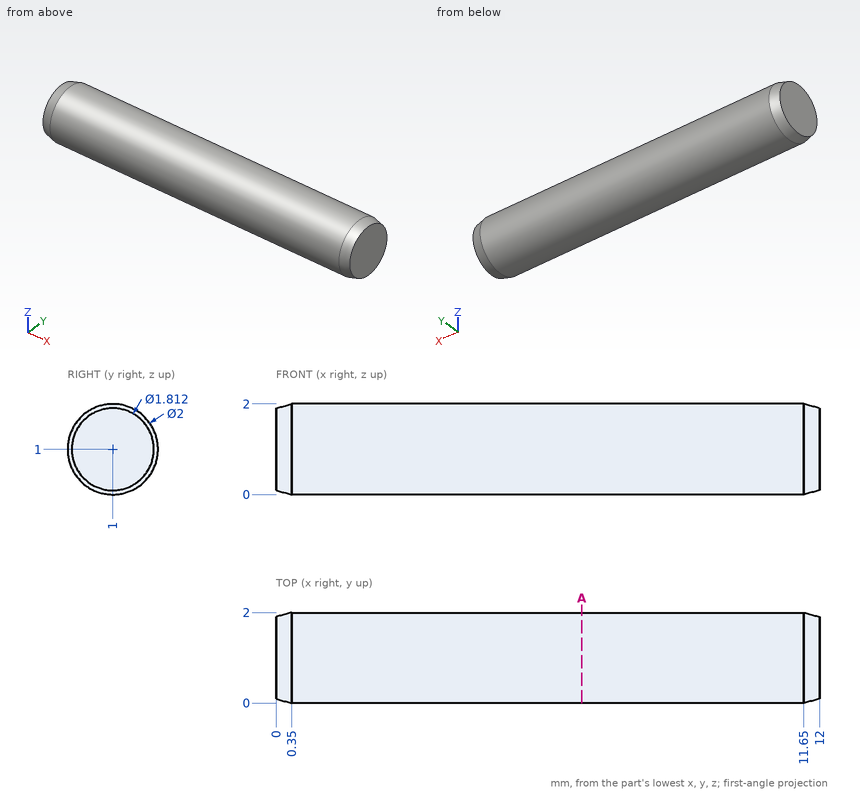
Geometry check sheet. Reference: drawing and pictorial views, mm from the part's lowest x, y, z. Give positions to 0.01 mm unless a question says otherwise; leave off trailing zeros. Order: outer loops, then holes, each group sorted by start corner. A loop starts at its lowest first (then second) coordinate and runs counter-clockwise, first axis right, second up. Notation, with made-up numbers: (2, 72) - (24, 72) arc R35 cw to (24, 105) - close; hole circle Ø5 at (68, 6.5). An arc over 180 degrees is marked (long way). Use one line per item in the form item = value.
1) Material ranges on probe 1 along Y at (x, z) = (7.75, 0.95); probe 2 along Z at (x, y) = (3.25, 1.4) (1 decimal), recorded low to high. Write a range as from..to.
Working result:
probe_1 = 0..2
probe_2 = 0.1..1.9
2) Sectioned sample at A-A (x = 6.75). Record the boundary of the cut face in (y, z).
Working result:
outline = circle Ø2 at (1, 1)
3) Depth check by flat-ended pin: pin 1 Ø1 at (x, y) = (5.5, 1.5) entering from -Z. Enter the tip coordinate at first touch or a pass-through.
Working result:
pin_1 = 0
